Can you work these out from the model? Positions are in its coordinate system, mm. Give positions to 0.01 mm unless a question says otherwise; leave off trailing zeros.
```python
from build123d import *

# Parameters (mm, degrees)
F0_R     = 7.5
F1_DEPTH = 3


with BuildPart() as f1:
    # F0 (on Front) → F1 (new body)
    with BuildSketch(Plane.XZ):
        Polygon((-409.777922, -62.315632), (-459.777922, -62.315632), (-459.777922, -162.315632), (390.222078, -162.315632), (390.222078, -62.315632), (340.222078, -62.315632), (340.222078, -112.315632), (336.222078, -112.315632), (336.222078, -62.315632), (-32.777922, -62.315632), (-32.777922, -112.315632), (-36.777922, -112.315632), (-36.777922, -62.315632), (-405.777922, -62.315632), (-405.777922, -112.315632), (-409.777922, -112.315632), align=None)
        with Locations((-359.777922, -112.315632)):
            Circle(F0_R, mode=Mode.SUBTRACT)
        with Locations((-294.777922, -112.315632)):
            Circle(F0_R, mode=Mode.SUBTRACT)
        with Locations((-229.777922, -112.315632)):
            Circle(F0_R, mode=Mode.SUBTRACT)
        with Locations((-164.777922, -112.315632)):
            Circle(F0_R, mode=Mode.SUBTRACT)
        with Locations((-99.777922, -112.315632)):
            Circle(F0_R, mode=Mode.SUBTRACT)
        with Locations((30.222078, -112.315632)):
            Circle(F0_R, mode=Mode.SUBTRACT)
        with Locations((95.222078, -112.315632)):
            Circle(F0_R, mode=Mode.SUBTRACT)
        with Locations((160.222078, -112.315632)):
            Circle(F0_R, mode=Mode.SUBTRACT)
        with Locations((225.222078, -112.315632)):
            Circle(F0_R, mode=Mode.SUBTRACT)
        with Locations((290.222078, -112.315632)):
            Circle(F0_R, mode=Mode.SUBTRACT)
    extrude(amount=F1_DEPTH)


solid = f1.part
```
1) For pin 1 Ø0.9 at (x, y) = (338, -1) entering from +Z; pin 2 Ø12 at (x, z) = (290.22, -112.32) entering from -Y, each with a flat end and sliding along its axis, tell me the tip position at first contact or that it passes through.
Values follow:
pin 1: stops at z = -112.32
pin 2: passes through
2) Suppose I cut it at A-A on y = -1.5. State how many separate pieces and enclosed holes the cut face has, plus the area to 3 significant figures.
Values follow:
separate pieces: 1
enclosed holes: 10
area: 82,600 mm2
3) If we mould it in two halves opening along Z, with no side actions, what happens to faces 1 (the face through (-41, -3, -112)), 2 (the face through (87.73, -1.48, -111.99))? For each: +Z half, -Z half, draft (parallel to the pull), parting line (faces both ways), or undercut.
Values follow:
face 1: draft
face 2: undercut
4) Please list where these lines run through material, in increasing order: L1, parallel to X at y = -2, z = -68; L2, parallel to Z at x = 219.5, y = -0.6; L3, parallel to Z at x = 23.5, y = -0.5.
Values follow:
L1: x = -459.78 to -409.78, -405.78 to -36.78, -32.78 to 336.22, 340.22 to 390.22
L2: z = -162.32 to -117.16, -107.47 to -62.32
L3: z = -162.32 to -115.64, -108.99 to -62.32
